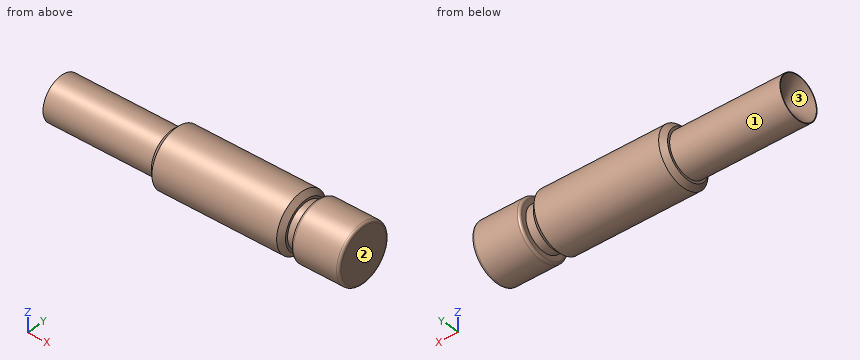
```python
from build123d import *

# Parameters (mm, degrees)
FILETE1_R     = 0.5
CHANFRO1_SIZE = 1


with BuildPart() as part:
    # Esboço1 → Revolução1 (revolve)
    with BuildSketch(Plane.XY, mode=Mode.PRIVATE) as revolu_o1_sk:
        Polygon((3.39980648, 0), (63, 0), (63, 6), (53, 6), (53, 4.5), (51, 4.5), (51, 6), (23, 6), (23, 4.5), (0, 4.5), (0, 4.356416698), align=None)
    revolve(revolu_o1_sk.sketch.rotate(Axis((3.39980648, 0, 0), (1, 0, 0)), 180), axis=Axis((3.39980648, 0, 0), (1, 0, 0)))

    # Filete1
    filete1_edges = [part.edges().sort_by_distance(p)[0] for p in [
        (53, 6, 0),
        (63, 6, 0),
    ]]
    fillet(filete1_edges, radius=FILETE1_R)

    # Chanfro1
    chanfro1_edges = [part.edges().sort_by_distance(p)[0] for p in [
        (51, 6, 0),
        (23, 6, 0),
    ]]
    chamfer(chanfro1_edges, length=CHANFRO1_SIZE)


solid = part.part
```
Check sheet for the modelled part. Datum: model origin and axes. Units: mm. Face numbers are marked on the shaded views. Round coordinates to 2 decimals unless told otherwise and drop trailing zeros. Loops run counter-clockwise (first coordinate to the right, second up) from the corner with the lowest first, then second, coordinate; pieces in that order, holes last. Notation, with made-up numbers: (26.25, -16.5) -> (45.25, -16.5) arc R17 cw to (45.25, -1.5) -> close; hole circle Ø4 at (48.5, -4.5). An arc over 180 degrees is marked (long way). Write item = value, one per line. Start each with the question number.
1) Release check for a two-part mould opening along Y. For the marked faces 1, 2 and 3 record: released by +Y, released by -Y, zero draft, split by the parting line, or undercut.
2) Gauge pin test, flat ends, axial feed: pin 1 Ø1.5 at (x, y) = (34.5, -4) entering from -Z; pin 2 Ø4 at (x, y) = (24, 3.5) entering from +Z; pin 3 Ø4 at (y, z) = (2, 1) entering from -X. Record the tip position at first contact, or that the pin passes through.
3) Thickness scan on probe 1 along X at (y, z) = (-4, 2.25); probe 2 along X at (y, z) = (4.5, -3); probe 3 along Y at (x, z) = (58, -2.5). Record the ranges inside material, lowest first.
4) Sectioned sample at B-B, the plane x = 39. Record the cut outline in (y, z), plus the area to 3 significant figures.
5) Sectioned sample at A-A, the plane x = 21.5. Record the cut outline in (y, z), plus the area to 3 significant figures.
Results are:
q1.face_1 = split by the parting line
q1.face_2 = zero draft
q1.face_3 = undercut
q2.pin_1 = -5.04
q2.pin_2 = 5.81
q2.pin_3 = 0.09
q3.probe_1 = 23 to 51, 53 to 63
q3.probe_2 = 23.41 to 50.59, 53 to 63
q3.probe_3 = -5.45 to 5.45
q4.outline = circle Ø12 at (0, 0)
q4.area = 113 mm^2
q5.outline = circle Ø9 at (0, 0)
q5.area = 63.6 mm^2
